Could you check a few things on this model? Use its own coordinates, in mm. Round coordinates to 2 decimals unless told otherwise and drop trailing zeros. Write each loop counter-clockwise with the first axis right and the second up, starting at its lowest first coordinate (ties: lowest second). Pieces come first, ordered by that corner, then holes. Notation, with made-up numbers: (-27, 63.5) -> (3, 63.5) arc R25 ccw to (3, 80.5) -> close; hole circle Ø10 at (61.5, -22). An arc over 180 degrees is marked (long way). Return JSON: item names as keys, results as strings.
from build123d import *

# Parameters (mm, degrees)
F1_DEPTH  = 1.5
F3_R      = 1.2
F4_DEPTH  = 4
F5_R      = 0.65
F6_DEPTH  = 25
F7_R      = 0.65
F8_DEPTH  = 25
F9_R      = 0.65
F10_DEPTH = 25
F12_DEPTH = 25
F2_R      = 2.6
F13_DEPTH = 25
F11_R     = 0.65
F14_DEPTH = 25


with BuildPart() as f1:
    # F0 (on Top) → F1 (new body)
    with BuildSketch(Plane.XY):
        with BuildLine():
            Line((8.771231, 7.214553), (-12.228769, 7.214553))
            ThreePointArc((-12.228769, 7.214553), (-12.935876, 6.92166), (-13.228769, 6.214553))
            Line((-13.228769, 6.214553), (-13.228769, -8.785447))
            ThreePointArc((-13.228769, -8.785447), (-12.935876, -9.492553), (-12.228769, -9.785447))
            Line((-12.228769, -9.785447), (8.771231, -9.785447))
            ThreePointArc((8.771231, -9.785447), (9.478338, -9.492553), (9.771231, -8.785447))
            Line((9.771231, -8.785447), (9.771231, 6.214553))
            ThreePointArc((9.771231, 6.214553), (9.478338, 6.92166), (8.771231, 7.214553))
        make_face()
    extrude(amount=F1_DEPTH)

    # F3 (on face) → F4 (cut)
    with BuildSketch(Plane.XY.offset(1.5)):
        with Locations((-5, -7)):
            Circle(F3_R)
        with Locations((5, -7)):
            Circle(F3_R)
    extrude(amount=-F4_DEPTH, mode=Mode.SUBTRACT)

    # F5 (on face) → F6 (cut)
    with BuildSketch(Plane.XY.offset(1.5)):
        with Locations((-7.628769, -7.7)):
            Circle(F5_R)
        with Locations((-7.628769, -5.177216)):
            Circle(F5_R)
        with Locations((-7.628769, -2.654431)):
            Circle(F5_R)
        with Locations((-4.458791, -2.654431)):
            Circle(F5_R)
    extrude(amount=-F6_DEPTH, mode=Mode.SUBTRACT)

    # F7 (on face) → F8 (cut)
    with BuildSketch(Plane.XY.offset(1.5)):
        with Locations((6.719702, 5.25)):
            Circle(F7_R)
        with Locations((6.719702, 1.130296)):
            Circle(F7_R)
        with Locations((6.719702, -3)):
            Circle(F7_R)
    extrude(amount=-F8_DEPTH, mode=Mode.SUBTRACT)

    # F9 (on face) → F10 (cut)
    with BuildSketch(Plane.XY.offset(1.5)):
        with Locations((-7.628769, 3.8)):
            Circle(F9_R)
        with Locations((-7.628769, 0.3)):
            Circle(F9_R)
    extrude(amount=-F10_DEPTH, mode=Mode.SUBTRACT)

    # F3 (on face) → F12 (cut)
    with BuildSketch(Plane.XY.offset(1.5)):
        with Locations((-5, -7)):
            Circle(F3_R)
        with Locations((5, -7)):
            Circle(F3_R)
    extrude(amount=-F12_DEPTH, mode=Mode.SUBTRACT)

    # F2 (on face) → F13 (cut)
    with BuildSketch(Plane.XY.offset(1.5)):
        with Locations((-0.228769, 0.214553)):
            Circle(F2_R)
    extrude(amount=-F13_DEPTH, mode=Mode.SUBTRACT)

    # F11 (on face) → F14 (cut)
    with BuildSketch(Plane.XY.offset(1.5)):
        with Locations((3, -3)):
            Circle(F11_R)
        with Locations((-3.3, 3.3)):
            Circle(F11_R)
    extrude(amount=-F14_DEPTH, mode=Mode.SUBTRACT)


solid = f1.part
1) I want a section at A-A, the plane x = 5. Please give me the cut outline in (y, z).
Return value:
{"outline": "(-9.79, 0) -> (-8.2, 0) -> (-8.2, 1.5) -> (-9.79, 1.5) -> close; (-5.8, 0) -> (7.21, 0) -> (7.21, 1.5) -> (-5.8, 1.5) -> close"}
2) If I drill on probe 1 along Y at (x, z) = (5, 0.4); probe 2 along X at (y, z) = (0.25, 1.2); probe 3 along X at (y, z) = (-7.25, 1.3), over which ranges is the centre line in solid material (lowest first)? Write a range as [from, to].
Return value:
{"probe 1": "[-9.79, -8.2], [-5.8, 7.21]", "probe 2": "[-13.23, -8.28], [-6.98, -2.83], [2.37, 9.77]", "probe 3": "[-13.23, -8.1], [-7.16, -6.17], [-3.83, 3.83], [6.17, 9.77]"}
3) Will this pin go through, and if not, where does the flat tip stop? pin 1 Ø1 at (x, y) = (6.72, 5.25) entering from +Z.
Return value:
{"pin 1": "through"}
4) I want a section at B-B, the plane y = -6.25. Please give me the cut outline in (x, z).
Return value:
{"outline": "(-13.23, 0) -> (-5.94, 0) -> (-5.94, 1.5) -> (-13.23, 1.5) -> close; (-4.06, 0) -> (4.06, 0) -> (4.06, 1.5) -> (-4.06, 1.5) -> close; (5.94, 0) -> (9.77, 0) -> (9.77, 1.5) -> (5.94, 1.5) -> close"}
5) Thinking about a two-plate mould opening in Y: for faces 1 (the face through (-12.944, -9.485, 0.74)), 2 (the face through (3.3, -3.577, 0.76)), 3 (the face through (-2, -3, 1.5)), which applies, pulls with the +Y half, pulls with the -Y half, needs draft (parallel to the pull), parting line crosses it, or undercut?
Return value:
{"face 1": "pulls with the -Y half", "face 2": "undercut", "face 3": "needs draft"}
6) I want a section at D-D, the plane x = -3.3. Please give me the cut outline in (y, z), and give its area (4 significant figures).
Return value:
{"outline": "(-9.79, 0) -> (2.65, 0) -> (2.65, 1.5) -> (-9.79, 1.5) -> close; (3.95, 0) -> (7.21, 0) -> (7.21, 1.5) -> (3.95, 1.5) -> close", "area": "23.55 mm²"}
7) I want a section at C-C, the plane y = -3. Please give me the cut outline in (x, z).
Return value:
{"outline": "(-13.23, 0) -> (-8.18, 0) -> (-8.18, 1.5) -> (-13.23, 1.5) -> close; (-7.08, 0) -> (-5.01, 0) -> (-5.01, 1.5) -> (-7.08, 1.5) -> close; (-3.91, 0) -> (2.35, 0) -> (2.35, 1.5) -> (-3.91, 1.5) -> close; (3.65, 0) -> (6.07, 0) -> (6.07, 1.5) -> (3.65, 1.5) -> close; (7.37, 0) -> (9.77, 0) -> (9.77, 1.5) -> (7.37, 1.5) -> close"}
